Design review of the part built by this model. Coordinates are the model's own, in mm. A direction names the side the tool comes from. Coordinates: 2 decimals unless noted, no trailing zeros. Write each loop counter-clockwise with the first axis right and the second up, starting at its lowest first coordinate (ties: lowest second). Pieces come first, ordered by that corner, then holes. Notation, with made-up numbers: (-20.75, -38) - (1.25, -38) arc R21 ccw to (1.25, -4) - close; hole circle Ø7 at (76.25, 61). An arc over 180 degrees is marked (long way). Answer as a JSON object with one key per item and string values.
```python
from build123d import *

# Parameters (mm, degrees)
SKETCH_W            = 83
SKETCH_H            = 94
PAD_DEPTH           = 15
SKETCH001_W         = 79
SKETCH001_H         = 10
POCKET_DEPTH        = 13
LINEARPATTERN_COUNT = 5
LINEARPATTERN_PITCH = 20
FILLET_R            = 3


with BuildPart() as part:
    # Sketch → Pad (new body)
    with BuildSketch(Plane.XY):
        Rectangle(SKETCH_W, SKETCH_H)
    extrude(amount=PAD_DEPTH)

    # Sketch001 (on Face6 of Pad) → Pocket (cut)
    with BuildSketch(Plane.XY.offset(15)):
        with Locations((0, 40)):
            Rectangle(SKETCH001_W, SKETCH001_H)
    pocket = extrude(amount=-POCKET_DEPTH, mode=Mode.SUBTRACT)

    # LinearPattern: Pocket ×5
    with Locations(*[(0, -i * LINEARPATTERN_PITCH, 0) for i in range(1, LINEARPATTERN_COUNT)]):
        add(pocket, mode=Mode.SUBTRACT)

    # Fillet
    fillet_edges = [part.edges().sort_by_distance(p)[0] for p in [
        (-41.5, 47, 7.5),
        (41.5, 47, 7.5),
        (-41.5, -47, 7.5),
        (41.5, -47, 7.5),
    ]]
    fillet(fillet_edges, radius=FILLET_R)


solid = part.part
```
(1) For pin 1 (3 mm diameter, centred on x = 13.5, y = 21, fed in from +Z); pin 2 (8 mm diameter, centred on x = 2, y = -18, fed in from +Z), all flat-tipped, find the tip position at first contact; note any pin that passes through.
Solved:
{"pin 1": "stops at z = 2", "pin 2": "stops at z = 15"}
(2) Take a section at B-B, the plane x = -33. Write out the cut boundary in (y, z), and give its area (3 significant figures).
Solved:
{"outline": "(-47, 0) - (47, 0) - (47, 15) - (45, 15) - (45, 2) - (35, 2) - (35, 15) - (25, 15) - (25, 2) - (15, 2) - (15, 15) - (5, 15) - (5, 2) - (-5, 2) - (-5, 15) - (-15, 15) - (-15, 2) - (-25, 2) - (-25, 15) - (-35, 15) - (-35, 2) - (-45, 2) - (-45, 15) - (-47, 15) - close", "area": "760 mm^2"}
(3) The part is to be moulded in two halves that separate along X. For faces 3 (the face through (-1, 35, 9)), 4 (the face through (40.6, -46.14, 7.6)), 5 (the face through (-1, -47, 7)), 6 (the face through (-1, -20, 2)), say which applies: pulls with the +X half, pulls with the -X half, needs draft (parallel to the pull), parting line crosses it, or undercut.
Solved:
{"face 3": "undercut", "face 4": "pulls with the +X half", "face 5": "needs draft", "face 6": "undercut"}
(4) Take a section at A-A, the plane z = 4.25. Write out the cut boundary in (x, y), and give its area (3 significant figures).
Solved:
{"outline": "(-41.5, -44) arc R3 ccw to (-38.5, -47) - (38.5, -47) arc R3 ccw to (41.5, -44) - (41.5, 44) arc R3 ccw to (38.5, 47) - (-38.5, 47) arc R3 ccw to (-41.5, 44) - close; hole (-39.5, -45) - (39.5, -45) - (39.5, -35) - (-39.5, -35) - close; hole (-39.5, -25) - (39.5, -25) - (39.5, -15) - (-39.5, -15) - close; hole (-39.5, -5) - (39.5, -5) - (39.5, 5) - (-39.5, 5) - close; hole (-39.5, 15) - (39.5, 15) - (39.5, 25) - (-39.5, 25) - close; hole (-39.5, 35) - (39.5, 35) - (39.5, 45) - (-39.5, 45) - close", "area": "3,840 mm^2"}
(5) To check wall thickness, follow line 1 (Y direction, x = -2, z = 5.75); line 2 (X direction, y = -35.5, z = 11.25); line 3 (Z direction, x = -34, y = -24.5). State the ranges of each line that lie inside material, in increasing order. Write a range as from..to.
Solved:
{"line 1": "y = -47..-45, -35..-25, -15..-5, 5..15, 25..35, 45..47", "line 2": "x = -41.5..-39.5, 39.5..41.5", "line 3": "z = 0..2"}
(6) Tool access review of faces 1 (the face through (-40.64, -46.1, 7.6)), 2 (the face through (-1, -40, 2)): name each direction out of +Z, -Z, +X, -X, +Y, -Y from which nothing blocks a thin tool from reaching the whole face with its end or side.
Solved:
{"face 1": "+Z, -Z, -X, -Y", "face 2": "+Z"}
